Study the drawing (mm; zero at the part's minimum x, y, z) and answer. Round coordinates to 2 decimals unless told otherwise and drop trailing zeros. Loops run counter-clockwise (first coordinate to the right, second up) from the corner with the lowest first, then second, coordinate; pieces in that order, holes last. Notation, with made-up numbers: (-38.5, 16) - (-22.5, 16) arc R9 ccw to (-22.5, 33) - close; hole circle Ø2 at (-11.75, 83.25). An arc over 180 degrees is marked (long way). Use CSV: the item, a comma, the result in double quotes. Start each with the question number.
1. Find section B-B (x = 19). Give the vertices of the cut face in (y, z).
2. Consider line 1 along Y through (x, z) = (13.5, 5); line 2 along X through (y, z) = (14, 4.85); line 3 along X through (y, z) = (53, 4.65). Determine where each line is inside the solid, lowest interval first.
3. Find section D-D (x = 25.5). Give the vertices of the cut face in (y, z).
4. Determine the mould class of the marked faces 1 and 2 for opening direction X: +X half, -X half, draft (parallel to the pull), parting line (faces both ways), or undercut.
5. Given pin 1 Ø1.5 at (x, y) = (10, 7) entering from +Z; pin 2 Ø0.8 at (y, z) = (53, 3) entering from -X; pin 3 Ø3 at (x, z) = (18.5, 3) entering from +Y, each flat-ended and moving along its own axis, determine where each tip first touches the part or whether it passes through.
6. Find section A-A (y = 14). Give the vertices of the cut face in (x, z).
7. Find section C-C (z = 3.8). State how many separate pieces and enclosed holes the cut face has, and give its area (3 significant figures).
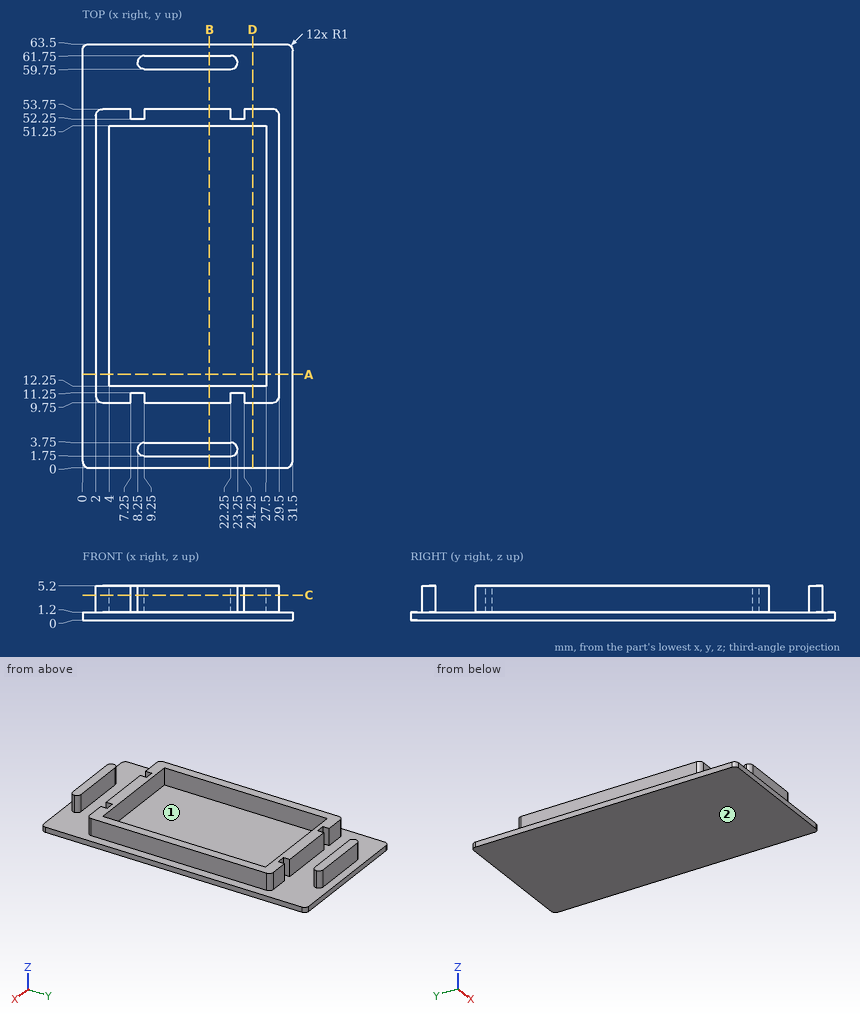
Filled sheet:
1,outline,"(0, 0) - (63.5, 0) - (63.5, 1.2) - (61.75, 1.2) - (61.75, 5.2) - (59.75, 5.2) - (59.75, 1.2) - (53.75, 1.2) - (53.75, 5.2) - (51.25, 5.2) - (51.25, 1.2) - (12.25, 1.2) - (12.25, 5.2) - (9.75, 5.2) - (9.75, 1.2) - (3.75, 1.2) - (3.75, 5.2) - (1.75, 5.2) - (1.75, 1.2) - (0, 1.2) - close"
2,line 1,"y = 1.75 to 3.75, 9.75 to 12.25, 51.25 to 53.75, 59.75 to 61.75"
2,line 2,"x = 2 to 4, 27.5 to 29.5"
2,line 3,"x = 2.03 to 7.25, 9.25 to 22.25, 24.25 to 29.47"
3,outline,"(0, 0) - (63.5, 0) - (63.5, 1.2) - (53.75, 1.2) - (53.75, 5.2) - (51.25, 5.2) - (51.25, 1.2) - (12.25, 1.2) - (12.25, 5.2) - (9.75, 5.2) - (9.75, 1.2) - (0, 1.2) - close"
4,face 1,"undercut"
4,face 2,"draft"
5,pin 1,"stops at z = 1.2"
5,pin 2,"stops at x = 2"
5,pin 3,"stops at y = 61.75"
6,outline,"(0, 0) - (31.5, 0) - (31.5, 1.2) - (29.5, 1.2) - (29.5, 5.2) - (27.5, 5.2) - (27.5, 1.2) - (4, 1.2) - (4, 5.2) - (2, 5.2) - (2, 1.2) - (0, 1.2) - close"
7,separate pieces,"3"
7,enclosed holes,"1"
7,area,"339 mm²"
